from build123d import *

# Parameters (mm, degrees)
SKETCH1_W           = 25.4
SKETCH1_H           = 25.4
SKETCH1_W_2         = 19.05
SKETCH1_H_2         = 19.05
BOSS_EXTRUDE1_DEPTH = 304.8
CUT_EXTRUDE1_DEPTH  = 307.120058147
SKETCH3_R           = 3.302
CUT_EXTRUDE2_DEPTH  = 307.120058147


with BuildPart() as part:
    # Sketch1 → Boss-Extrude1 (new body)
    with BuildSketch(Plane.XY):
        Rectangle(SKETCH1_W, SKETCH1_H)
        Rectangle(SKETCH1_W_2, SKETCH1_H_2, mode=Mode.SUBTRACT)
    extrude(amount=BOSS_EXTRUDE1_DEPTH)

    # Sketch2 → Cut-Extrude1 (cut, through all)
    with BuildSketch(Plane(origin=(12.7, 0, 0), x_dir=(0, 0, -1), z_dir=(1, 0, 0))):
        Polygon((0, 12.7), (0, -12.7), (-25.4, 12.7), align=None)
    extrude(amount=-CUT_EXTRUDE1_DEPTH, mode=Mode.SUBTRACT)

    # Sketch3 → Cut-Extrude2 (cut, through all)
    with BuildSketch(Plane(origin=(0, 12.7, 0), x_dir=(1, 0, 0), z_dir=(0, 1, 0))):
        with Locations(Location((0, -76.2, 0), (0, 0, 180))):
            Circle(SKETCH3_R)
    extrude(amount=-CUT_EXTRUDE2_DEPTH, mode=Mode.SUBTRACT)


solid = part.part
Could you check a few things on this model? Use its own coordinates, in mm. A direction names the side the tool comes from. Give positions to 0.01 mm unless a question says otherwise; leave off trailing zeros. Order: outer loops, then holes, each group sorted by start corner. A loop starts at its lowest first (then second) coordinate and runs counter-clockwise, first axis right, second up. Notation, with made-up numbers: (36.5, 87.5) - (85.5, 87.5) arc R33 ccw to (85.5, 125.5) - close; hole circle Ø2 at (-6.75, 31.5). An arc over 180 degrees is marked (long way). Return JSON: item names as keys, results as strings. Group by question number.
Q1. Please list where these lines run through material, in increasing order: line 1 along Y through (x, z) = (1.5, 153.5) (3 decimals); line 2 along Z through (x, y) = (-10, 9.5). Write a range as [from, to].
Q2. Will this pin go through, and if not, where does the flat tip stop? pin 1 Ø10 at (x, y) = (0.5, -6.5) entering from -Z.
Q3. Which directions (+Z, -Z, +X, -X, +Y, -Y) give clear straight access to the entire face, cutting with the end or side of a thin tool? Please do faces 4 (the face through (-11.1, -0.2, 12.5)), 5 (the face through (-9.525, 0, 152)).
Q4. Suppose I cut it at A-A, the plane z = 76.2. Please give me the cut outline in (x, y) (3 decimals).
Q5. Suppose I cut it at D-D, the plane z = 129.5. Please give me the cut outline in (x, y) (3 decimals), and give its area (3 significant figures).
Q6. Suppose I cut it at B-B, the plane x = 0. Please give me the cut outline in (y, z) (3 decimals).
Q7. Thinking about a two-plate mould opening in X: for faces 1 (the face through (-12.7, 0, 150)), 2 (the face through (0.716, 11.135, 72.977)), 3 (the face through (11, 0, 304.8)), which applies, pulls with the +X half, pulls with the -X half, needs draft (parallel to the pull), parting line crosses it, or undercut?
Q8. Suppose I cut it at C-C, the plane y = 3. Please give me the cut outline in (x, z) (3 decimals).
Resolved:
{
 "1": {"line 1": "y = [-12.7, -9.525], [9.525, 12.7]", "line 2": "z = [22.2, 304.8]"},
 "2": {"pin 1": "stops at z = 1.2"},
 "3": {"face 4": "-Z, +X, -X, +Y", "face 5": "+Z, -Z"},
 "4": {"outline": "(-12.7, -12.7) - (-3.302, -12.7) - (-3.302, -9.525) - (-9.525, -9.525) - (-9.525, 9.525) - (-3.302, 9.525) - (-3.302, 12.7) - (-12.7, 12.7) - close; (3.302, -12.7) - (12.7, -12.7) - (12.7, 12.7) - (3.302, 12.7) - (3.302, 9.525) - (9.525, 9.525) - (9.525, -9.525) - (3.302, -9.525) - close"},
 "5": {"outline": "(-12.7, -12.7) - (12.7, -12.7) - (12.7, 12.7) - (-12.7, 12.7) - close; hole (-9.525, -9.525) - (9.525, -9.525) - (9.525, 9.525) - (-9.525, 9.525) - close", "area": "282 mm2"},
 "6": {"outline": "(-12.7, 0) - (-9.525, 3.175) - (-9.525, 72.898) - (-12.7, 72.898) - close; (-12.7, 79.502) - (-9.525, 79.502) - (-9.525, 304.8) - (-12.7, 304.8) - close; (9.525, 22.225) - (12.7, 25.4) - (12.7, 72.898) - (9.525, 72.898) - close; (9.525, 79.502) - (12.7, 79.502) - (12.7, 304.8) - (9.525, 304.8) - close"},
 "7": {"face 1": "pulls with the -X half", "face 2": "undercut", "face 3": "needs draft"},
 "8": {"outline": "(-12.7, 15.7) - (-9.525, 15.7) - (-9.525, 304.8) - (-12.7, 304.8) - close; (9.525, 15.7) - (12.7, 15.7) - (12.7, 304.8) - (9.525, 304.8) - close"}
}
